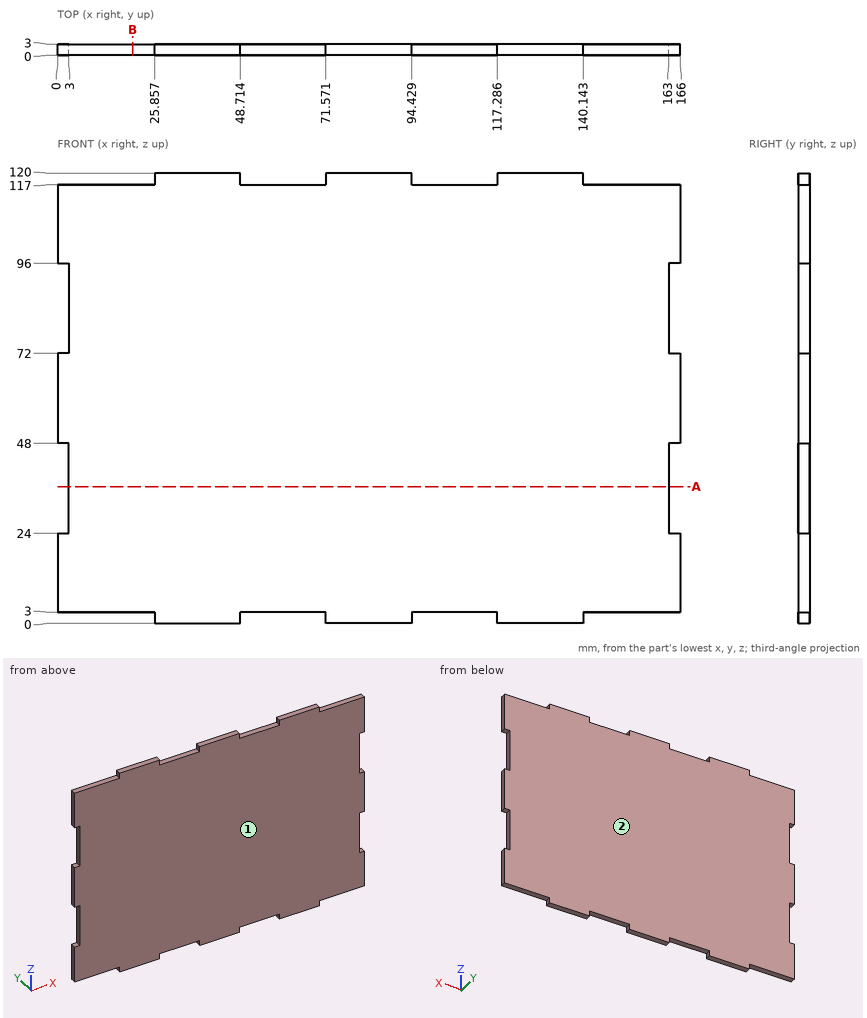
Can you work these out from the drawing? Everything is in mm from the part's minimum corner. Coordinates: 2 decimals unless noted, no trailing zeros. Write each loop counter-clockwise with the first axis right and the second up, starting at its lowest first coordinate (ties: lowest second). Pieces come first, ordered by that corner, then holes. Notation, with made-up numbers: (-7.5, 11.5) -> (28.5, 11.5) arc R30 cw to (28.5, 49.5) -> close; hole circle Ø4 at (-7, 32.25). An arc over 180 degrees is marked (long way). Return JSON: item names as keys, results as strings.
(1) I'm going to push flat-ended pins straight in: pin 1 (1 mm diameter, centred on x = 112, z = 88, fed in from -Y); pin 2 (1.5 mm diameter, centred on x = 143.5, y = 2, fed in from +Z); pin 3 (0.9 mm diameter, centred on y = 2, z = 119, fed in from -X); pin 4 (0.9 mm diameter, centred on y = 2, z = 2, fed in from +X). Where does each tip first touch, or does it pass through?
Numbers:
{"pin 1": "stops at y = 0", "pin 2": "stops at z = 117", "pin 3": "stops at x = 25.86", "pin 4": "stops at x = 140.14"}
(2) I need wall thicknesses on L1, parallel to Z at x = 66, y = 2.3; L2, parallel to X at y = 0.4, z = 90.5. Which ranges of each line are inside material? Lowest first, please.
Numbers:
{"L1": "z = 3 to 117", "L2": "x = 3 to 163"}
(3) Imagine slicing it at A-A, the plane z = 36.5. Please give me the cut outline in (x, y), then the cut area to 3 significant figures.
Numbers:
{"outline": "(3, 0) -> (163, 0) -> (163, 3) -> (3, 3) -> close", "area": "480 mm2"}
(4) Imagine slicing it at B-B, the plane x = 20. Please give me the cut outline in (y, z), then the cut area to 3 significant figures.
Numbers:
{"outline": "(0, 3) -> (3, 3) -> (3, 117) -> (0, 117) -> close", "area": "342 mm2"}
(5) We'd pull the mould along Y, two halves only. Please class the marked faces 1 and 2: +Y half, -Y half, draft (parallel to the pull), parting line (faces both ways), or undercut.
Numbers:
{"face 1": "-Y half", "face 2": "+Y half"}
